For this review, take the finished solid that the model builds, in its own axes (mm). Coordinates: 2 decimals unless noted, no trailing zeros. Loops run counter-clockwise (first coordinate to the right, second up) from the corner with the lowest first, then second, coordinate; pieces in that order, holes last. Notation, with made-up numbers: M 4,-27.75 L 16,-27.75 A22 ccw 16,-21.75 Z; hole C -0.75,73.25 d9. An arc over 180 degrees is marked long. Put each result on its own line as item: value.
```python
from build123d import *

# Parameters (mm, degrees)
SKETCH_1_R          = 0.1625092
SKETCH_1_R_2        = 0.2249932
SKETCH_1_R_3        = 0.1124966
EXTRUDE_1_DEPTH     = 1.5
SKETCH_2_R          = 1.25
CUT_EXTRUDE_1_DEPTH = 171.139217701


with BuildPart() as part:
    # 草图1 → 凸台-拉伸1 (new body)
    with BuildSketch(Plane(origin=(0, 0, 0), x_dir=(1, 0, 0), z_dir=(0, 1, 0))):
        Polygon((139.065, 95.25), (120.015, 95.25), (118.11, 93.345), (118.11, 59.69), (121.92, 55.88), (137.16, 55.88), (140.97, 59.69), (140.97, 93.345), align=None)
        with Locations(Location((126.65202, 89.94902, 0), (0, 0, 270))):
            Circle(SKETCH_1_R, mode=Mode.SUBTRACT)
        with Locations(Location((132.42798, 89.94902, 0), (0, 0, 270))):
            Circle(SKETCH_1_R, mode=Mode.SUBTRACT)
        with Locations(Location((133.35, 58.166, 0), (0, 0, 270))):
            Circle(SKETCH_1_R_2, mode=Mode.SUBTRACT)
        with Locations(Location((130.81, 58.166, 0), (0, 0, 270))):
            Circle(SKETCH_1_R_2, mode=Mode.SUBTRACT)
        with Locations(Location((128.27, 58.166, 0), (0, 0, 270))):
            Circle(SKETCH_1_R_2, mode=Mode.SUBTRACT)
        with Locations(Location((125.73, 58.166, 0), (0, 0, 270))):
            Circle(SKETCH_1_R_2, mode=Mode.SUBTRACT)
        with Locations(Location((139.192, 68.58, 0), (0, 0, 270))):
            Circle(SKETCH_1_R_2, mode=Mode.SUBTRACT)
        with Locations(Location((139.192, 66.04, 0), (0, 0, 270))):
            Circle(SKETCH_1_R_2, mode=Mode.SUBTRACT)
        with Locations(Location((139.192, 63.5, 0), (0, 0, 270))):
            Circle(SKETCH_1_R_2, mode=Mode.SUBTRACT)
        with Locations(Location((139.192, 60.96, 0), (0, 0, 270))):
            Circle(SKETCH_1_R_2, mode=Mode.SUBTRACT)
        with Locations(Location((119.507, 77.724, 0), (0, 0, 270))):
            Circle(SKETCH_1_R_3, mode=Mode.SUBTRACT)
        with Locations(Location((119.507, 76.454, 0), (0, 0, 270))):
            Circle(SKETCH_1_R_3, mode=Mode.SUBTRACT)
        with Locations(Location((119.507, 73.914, 0), (0, 0, 270))):
            Circle(SKETCH_1_R_3, mode=Mode.SUBTRACT)
        with Locations(Location((119.507, 75.184, 0), (0, 0, 270))):
            Circle(SKETCH_1_R_3, mode=Mode.SUBTRACT)
    extrude(amount=EXTRUDE_1_DEPTH)

    # 草图2 → 切除-拉伸1 (cut, through all)
    with BuildSketch(Plane(origin=(0, 1.5, 0), x_dir=(1, 0, 0), z_dir=(0, 1, 0))):
        with Locations(Location((129.667, 82.804, 0), (0, 0, 270))):
            Circle(SKETCH_2_R)
    extrude(amount=-CUT_EXTRUDE_1_DEPTH, mode=Mode.SUBTRACT)


solid = part.part
```
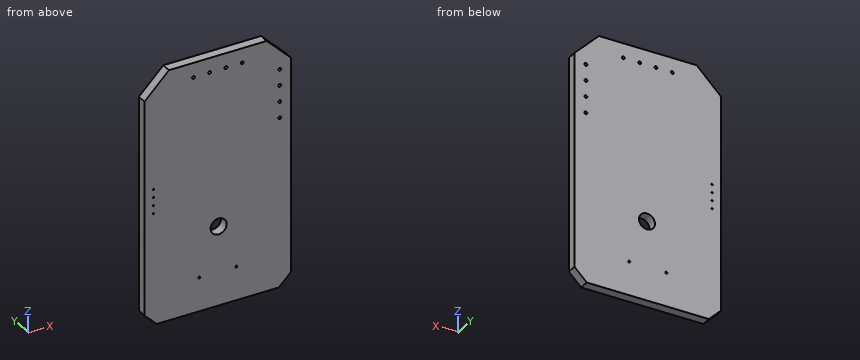
(1) Add section B-B (x = 121.25). Write out the cut boundary in (y, z).
Determined:
outline: M 0,-95.25 L 1.5,-95.25 L 1.5,-56.55 L 0,-56.55 Z
(2) Add section A-A (y = 0.6). State how many separate pieces and enclosed holes the cut face has, plus the area to 3 significant figures.
Determined:
separate pieces: 1
enclosed holes: 15
area: 875 mm^2
(3) For pin 1 (6 mm diameter, centred on x = 124.5, z = -80, fed in from -Y); pin 2 (1.5 mm diameter, centred on x = 129.667, z = -82.804, fed in from +Y), all flat-tipped, find the tip position at first contact; note any pin that passes through.
Determined:
pin 1: stops at y = 0
pin 2: passes through
(4) Wall thickness on line 1 along Z through (x, y) = (125.75, 0.8); line 2 along X through (y, z) = (1.3, -58); line 3 along X through (y, z) = (1, -66.04): over which ranges is each line inside the solid? List them lowest first. Write a range as [from, to].
Determined:
line 1: z = [-95.25, -58.39], [-57.94, -55.88]
line 2: x = [119.8, 125.58], [125.88, 128.12], [128.42, 130.66], [130.96, 133.2], [133.5, 139.28]
line 3: x = [118.11, 138.97], [139.42, 140.97]
